Here's how the part is built. I have some questions about the finished solid (model axes, mm). Face numbers are marked on the shaded views. A direction names the side the tool comes from. Give positions to 0.01 mm unless a question says otherwise; leave off trailing zeros. Loops run counter-clockwise (first coordinate to the right, second up) from the corner with the lowest first, then second, coordinate; pieces in that order, holes last.
Q1. I need wall thicknesses on probe 1 along Y at (x, z) = (-25, 0.5); probe 2 along X at (y, z) = (-5.5, -5); probe 3 along X at (y, z) = (4, -11). Which ranges of each line are inside material? Lowest first, please.
Q2. For the marked faces 1 and 2, which set-ups out of +Z, -Z, +X, -X, +Y, -Y let a thin tool reach every point of the face, with its end or its side?
Q3. I'm going to push flat-ended pins straight in: P1, Ø0.6, axis at y = -8.5, z = -5, coming from the -X side; P2, Ø2, axis at x = -8, z = 9.5, coming from the +Y side; P3, Ø4, axis at x = -24, y = -8.5, coming from the -Z side. Where does each tip first touch, or does it pass through?
Q4. Suppose I cut it at A-A (z = 0). List the corners of the cut face in (x, y) for me.
Q5. Suppose I cut it at B-B (x = -26). List the corners of the cut face in (y, z) for me.
Q6. Suppose I cut it at C-C (x = 5.5). List the corners of the cut face in (y, z) for me, and give its area (3 significant figures).
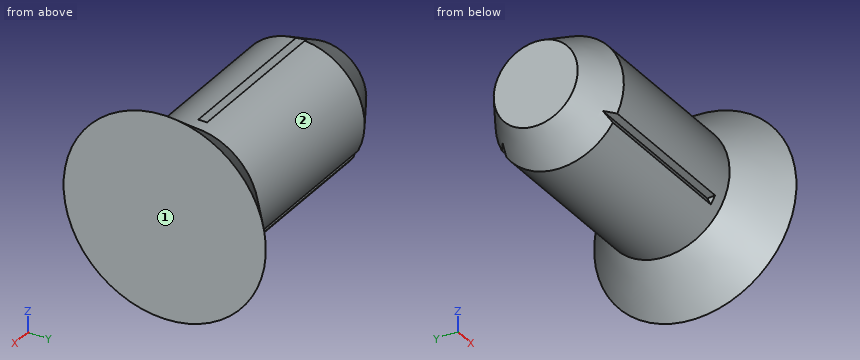
```python
from build123d import *

# Parameters (mm, degrees)
CUT_EXTRUDE1_DEPTH = 30.506454095
CIRPATTERN1_COUNT  = 3


with BuildPart() as part:
    # Sketch1 → Base-Revolve (revolve)
    with BuildSketch(Plane.XY, mode=Mode.PRIVATE) as base_revolve_sk:
        Polygon((-32.506454106, 0), (-32.506454106, 6.535898385), (-26.506454106, 10), (0, 10), (7.493545894, 15.75), (7.493545894, 0), align=None)
    revolve(base_revolve_sk.sketch.rotate(Axis((-40, 0, 0), (1, 0, 0)), 90), axis=Axis((-40, 0, 0), (1, 0, 0)))

    # Sketch2 → Cut-Extrude1 (cut)
    with BuildSketch(Plane.ZY.offset(32.506454106)):
        Polygon((9, 0), (10, 0.700207538), (10, -0.700207538), align=None)
    cut_extrude1 = extrude(amount=-CUT_EXTRUDE1_DEPTH, mode=Mode.SUBTRACT)

    # CirPattern1: Cut-Extrude1 ×3 about axis
    cirpattern1_axis = Axis((0, 0, 0), (1, 0, 0))
    for i in range(1, CIRPATTERN1_COUNT):
        add(cut_extrude1.rotate(cirpattern1_axis, i * 360 / CIRPATTERN1_COUNT), mode=Mode.SUBTRACT)


solid = part.part
```
Solutions:
1. probe 1: y = -9.99 to 9.99
1. probe 2: x = -30.95 to 7.49
1. probe 3: x = 2.22 to 7.49
2. face 1: +Z, -Z, +X, +Y, -Y
2. face 2: -X
3. P1: stops at x = -2
3. P2: stops at y = 5.27
3. P3: stops at z = -7.6
4. outline: (-32.51, -6.54) - (-26.51, -10) - (0, -10) - (7.49, -15.75) - (7.49, 15.75) - (0, 10) - (-26.51, 10) - (-32.51, 6.54) - close
5. outline: (-8.98, -4.4) - (-7.79, -4.5) - (-8.3, -5.58) arc R10 ccw to (8.3, -5.58) - (7.79, -4.5) - (8.98, -4.4) arc R10 ccw to (0.68, 9.98) - (0, 9) - (-0.68, 9.98) arc R10 ccw to start
6. outline: circle Ø28.44 at (0, 0)
6. area: 635 mm2
